```python
from build123d import *

# Parameters (mm, degrees)
SKETCH1_R           = 50
SKETCH1_R_2         = 30
SKETCH1_R_3         = 1.75
BOSS_EXTRUDE1_DEPTH = 3
CUT_EXTRUDE1_DEPTH  = 14
FILLET1_R           = 3


with BuildPart() as part:
    # Sketch1 → Boss-Extrude1 (new body)
    with BuildSketch(Plane(origin=(0, 0, 0), x_dir=(1, 0, 0), z_dir=(0, 1, 0))):
        with Locations(Location((0, 0, 0), (0, 0, 270))):
            Circle(SKETCH1_R)
        with Locations(Location((0, 0, 0), (0, 0, 270))):
            Circle(SKETCH1_R_2, mode=Mode.SUBTRACT)
        with Locations(Location((0, 45, 0), (0, 0, 270))):
            Circle(SKETCH1_R_3, mode=Mode.SUBTRACT)
        with Locations(Location((38.97114317, -22.5, 0), (0, 0, 270))):
            Circle(SKETCH1_R_3, mode=Mode.SUBTRACT)
        with Locations(Location((-38.97114317, -22.5, 0), (0, 0, 270))):
            Circle(SKETCH1_R_3, mode=Mode.SUBTRACT)
    extrude(amount=BOSS_EXTRUDE1_DEPTH)

    # Sketch2 → Cut-Extrude1 (cut)
    with BuildSketch(Plane(origin=(0, 3, 0), x_dir=(1, 0, 0), z_dir=(0, 1, 0))):
        Polygon((0, 0), (-50, -50), (50, -50), align=None)
    extrude(amount=-CUT_EXTRUDE1_DEPTH, mode=Mode.SUBTRACT)

    # Fillet1
    fillet1_edges = [part.edges().sort_by_distance(p)[0] for p in [
        (-21.213203436, 1.5, 21.213203436),
        (21.213203436, 1.5, 21.213203436),
        (35.355339059, 1.5, 35.355339059),
        (-35.355339059, 1.5, 35.355339059),
    ]]
    fillet(fillet1_edges, radius=FILLET1_R)


solid = part.part
```
Could you check a few things on this model? Use its own coordinates, in mm. A direction names the side the tool comes from. Coordinates: 2 decimals unless noted, no trailing zeros. Order: outer loops, then holes, each group sorted by start corner. A loop starts at its lowest first (then second) coordinate and runs counter-clockwise, first axis right, second up. Notation, with made-up numbers: M 65.5,82.25 L 116.5,82.25 A27 cw 116.5,100.25 Z; hole C -17,-18.75 d7. An arc over 180 degrees is marked long. Use a Markdown table: item, result. Add a question column.
Q1. I want a section at A-A on z = 0. List the corners of the cut face in (x, y) for me.
Q2. We'd pull the mould along X, two halves only. Please class faces 4 (the cylindrical face through (0.951, 1.479, -29.985)), 5 (the flat face through (1, 3, -37)), 6 (the cylindrical face through (1.604, 1.479, -49.974)): pulls with the +X half, pulls with the -X half, needs draft (parallel to the pull), parting line crosses it, or undercut.
Q3. I'm going to push flat-ended pins straight in: pin 1 (1.5 mm diameter, centred on y = 2.5, z = -27, fed in from -X); pin 2 (1.5 mm diameter, centred on x = -39.5, y = 2.5, fed in from -Z). Where does each tip first touch, or does it pass through?
Q4. If I drill on L1, parallel to X at y = 1.65, z = 22.5; L2, parallel to Z at x = 23, y = 2.45; L3, parallel to Z at x = 27, y = 1.5, over which ranges is the centre line in solid material (lowest first)?
Q5. Which directions (+Z, -Z, +X, -X, +Y, -Y) give clear straight access to the entire face, cutting with the end or side of a thin tool? Please do faces 1 (the cylindrical face through (-22.364, 1.479, 21.284)), 2 (the flat face through (1, 0, -37)), 3 (the flat face through (28, 2, 28)).
Q6. I want a section at B-B on x = 0. List the corners of the cut face in (y, z) for me, then the cut area to 3 significant figures.
Q7. I want a section at C-C on y = 0.75. List the corners of the cut face in (x, z) for me, then the cut area to 3 significant figures.
Q8. I want a section at D-D on x = 43. List the corners of the cut face in (y, z) for me, then the cut area to 3 significant figures.
Checked values:
| question | item | result |
|---|---|---|
| 1 | outline | M -50,0 L -30,0 L -30,3 L -50,3 Z; M 30,0 L 50,0 L 50,3 L 30,3 Z |
| 2 | face 4 | undercut |
| 2 | face 5 | needs draft |
| 2 | face 6 | parting line crosses it |
| 3 | pin 1 | x = -42.56 |
| 3 | pin 2 | z = -31.6 |
| 4 | L1 | -44.65 to -40.72, -37.22 to -22.7, 22.7 to 37.22, 40.72 to 44.65 |
| 4 | L2 | -44.4 to -19.26, 19.26 to 22.97 |
| 4 | L3 | -42.08 to -13.08, 13.08 to 27 |
| 5 | face 1 | +Y, -Y |
| 5 | face 2 | +Z, -Z, +X, -X, -Y |
| 5 | face 3 | +Z, +Y, -Y |
| 6 | outline | M 0,-50 L 3,-50 L 3,-46.75 L 0,-46.75 Z; M 0,-43.25 L 3,-43.25 L 3,-30 L 0,-30 Z |
| 6 | area | 49.5 mm² |
| 7 | outline | M -37.54,33.03 A50 ccw long 37.54,33.03 A3 ccw 33.17,33.17 L 23.24,23.24 A3 ccw 23.05,19.2 A30 cw long -23.05,19.2 A3 ccw -23.24,23.24 L -33.17,33.17 A3 ccw Z; hole C -38.97,22.5 d3.5; hole C 0,-45 d3.5; hole C 38.97,22.5 d3.5 |
| 7 | area | 3,730 mm² |
| 8 | outline | M 0,-25.51 L 3,-25.51 L 3,25.51 L 0,25.51 Z |
| 8 | area | 153 mm² |
